Job drawing, mm, ordinate dimensions from the low corner. One solid piece. Round coordinates to 2 decimals unless told otherwise and drop trailing zeros. Order: outer loops, then holes, each group sorted by start corner. A loop starts at its lowest first (then second) coordinate and runs counter-clockwise, first axis right, second up. Notation, with made-up numbers: (60, 54) -> (119, 54) arc R26 ccw to (119, 76) -> close; hole circle Ø6 at (76, 11.5). An arc over 180 degrees is marked (long way). Write item = value, one per line.
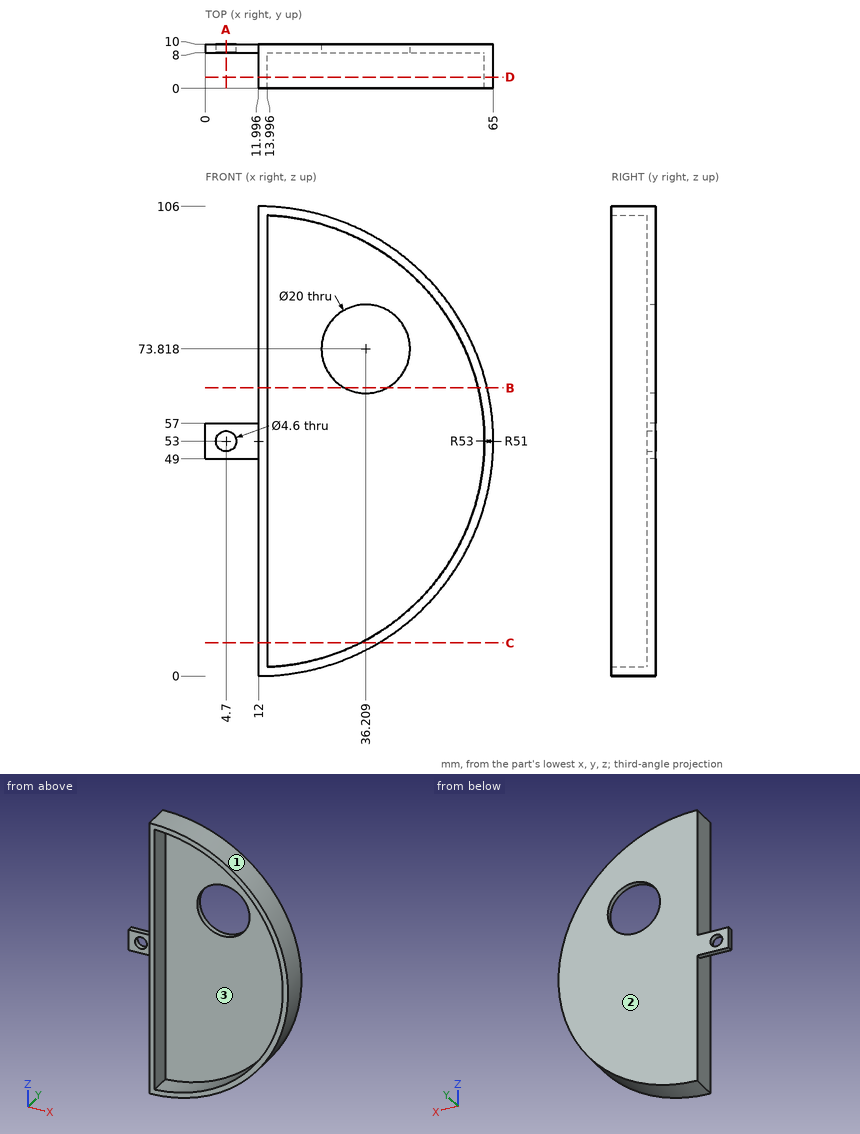
Q1. Mould opens along Z. For the marked faces 1, 2 and 3 say: released by +Z, released by -Z, zero draft, split by the parting line, or undercut.
Check values:
face_1 = split by the parting line
face_2 = zero draft
face_3 = undercut
Q2. Cut at D-D, the plane y = 2.5. List the corners of the cut face in (x, z).
Check values:
outline = (12, 0) arc R53 ccw to (12, 106) -> close; hole (14, 2.04) arc R51 ccw to (14, 103.96) -> close
Q3. Flat gauge pins, fed straight in: pin 1 (6.5 mm diameter, centred on x = 6, z = 52, fed in from -Y); pin 2 (1.6 mm diameter, centred on x = 4, y = 9, fed in from +Z); pin 3 (2 mm diameter, centred on x = 53.5, z = 86.5, fed in from +Y); pin 4 (5 mm diameter, centred on x = 33.5, y = 2, fed in from +Z). Where does each tip first touch, or does it go through?
Check values:
pin_1 = 8
pin_2 = 57
pin_3 = 10
pin_4 = 102.48
Q4. Cut at C-C, the plane z = 7.5. List the corners of the cut face in (x, y).
Check values:
outline = (12, 0) -> (14, 0) -> (14, 8) -> (35.04, 8) -> (35.04, 0) -> (39.18, 0) -> (39.18, 10) -> (12, 10) -> close
Q5. Probe probe 1 along Z at (x, y) = (4.7, 8.65); probe 2 along X at (y, z) = (7, 52); probe 3 along Y at (x, z) = (47.5, 17). List the from-to ranges inside material, lowest first.
Check values:
probe_1 = 49 to 50.7, 55.3 to 57
probe_2 = 12 to 14, 62.99 to 64.99
probe_3 = 8 to 10
Q6. Cut at A-A, the plane x = 4.7. List the corners of the cut face in (y, z).
Check values:
outline = (8, 49) -> (10, 49) -> (10, 50.7) -> (8, 50.7) -> close; (8, 55.3) -> (10, 55.3) -> (10, 57) -> (8, 57) -> close
Q7. Cut at B-B, the plane z = 65. List the corners of the cut face in (x, y) (1 decimal), and give its area (3 significant figures).
Check values:
outline = (12, 0) -> (14, 0) -> (14, 8) -> (31.5, 8) -> (31.5, 10) -> (12, 10) -> close; (40.9, 8) -> (61.6, 8) -> (61.6, 0) -> (63.6, 0) -> (63.6, 10) -> (40.9, 10) -> close
area = 117 mm²
